Verification items for the finished model (mm, model axes). A direction names the side the tool comes from. Give positions to 0.01 mm unless a question says otherwise; leave off trailing zeros. Write each loop counter-clockwise with the first axis right and the second up, starting at its lowest first coordinate (ties: lowest second). Pieces come first, ordered by that corner, then holes. Notation, with made-up numbers: (79, 89) -> (121, 89) arc R30 cw to (121, 114) -> close; hole circle Ø10 at (8.25, 35.25). An arc over 180 degrees is marked (long way). Answer as CSV lines item,"result". Start each with the question number.
1) Material ranges on L1, parallel to Y at x = 5.5, z = 2.6; L2, parallel to Y at x = 5.5, z = 2.45; L3, parallel to Z at x = -4.5, y = 9, recorded low to high.
2) Sectioned sample at C-C on y = 14. Record the cut outline in (x, z), and give its area (3 significant figures).
3) Mould release check, pull along Y, two halves, no side actions. Record for faces 4 (the flat face through (5, 33, 1)), 5 (the flat face through (-4, 36, 1)), 6 (the flat face through (12, -11.5, 1)), 7 (the flat face through (6.25, 10, 1)): released by +Y, released by -Y, zero draft, split by the parting line, or undercut.
4) Gauge pin test, flat ends, axial feed: pin 1 Ø3.5 at (y, z) = (39.5, 1.5) entering from +X; pin 2 Ø12 at (x, y) = (9.5, 10.5) entering from +Z; pin 3 Ø2 at (y, z) = (2, 3.5) entering from +X; pin 4 Ø3 at (x, y) = (-2.5, 35) entering from -Z. Record the tip position at first contact, or that the pin passes through.
5) Tool access check on faces 1 (the flat face through (4, 42, 1)), 2 (the flat face through (6, 40, 2)), 3 (the cylindrical face through (6.63, -20.48, 2.01)). Record the directions out of +Z, -Z, +X, -X, +Y, -Y that give a thin tool (end or side, any length) a straight path to the whole face; none if there is none.
6) Sectioned sample at B-B on x = 10.75. Record the cut outline in (y, z), and give its area (3 significant figures).
7) Sectioned sample at A-A on y = -22.25. Record the cut outline in (x, z), and give its area (3 significant figures).
```python
from build123d import *

# Parameters (mm, degrees)
PAD_DEPTH    = 3
SKETCH001_R  = 1.5
PAD001_DEPTH = 6
SKETCH002_R  = 2.1
POCKET_DEPTH = 2
SKETCH003_R  = 3
PAD002_DEPTH = 3
FILLET_R     = 2.75


with BuildPart() as part:
    # Sketch → Pad (new body)
    with BuildSketch(Plane.XY):
        Polygon((-6.25, 33), (-6.25, -33), (17.25, -33), (17.25, -11.5), (6.25, -11.5), (6.25, 33), (4, 33), (4, 43), (-4, 43), (-4, 33), align=None)
    extrude(amount=PAD_DEPTH)

    # Sketch001 → Pad001 (join, symmetric)
    with BuildSketch(Plane.YZ):
        with Locations((40, 1.5)):
            Circle(SKETCH001_R)
    extrude(amount=PAD001_DEPTH, both=True)

    # Sketch002 (on Face5 of Pad001) → Pocket (cut)
    with BuildSketch(Plane.XY.offset(3)):
        with Locations((5.5, -22.25)):
            Circle(SKETCH002_R)
    extrude(amount=-POCKET_DEPTH, mode=Mode.SUBTRACT)

    # Sketch003 (on Face5 of Pocket) → Pad002 (join)
    with BuildSketch(Plane.XY.offset(3)):
        with Locations((0, 23)):
            Circle(SKETCH003_R)
    extrude(amount=PAD002_DEPTH)

    # Fillet
    fillet_edges = [part.edges().sort_by_distance(p)[0] for p in [
        (-3, 23, 6),
    ]]
    fillet(fillet_edges, radius=FILLET_R)


solid = part.part
```
Ans:
1,L1,"y = -33 to -24.35, -20.15 to 33, 38.98 to 41.02"
1,L2,"y = -33 to -24.35, -20.15 to 33, 38.84 to 41.16"
1,L3,"z = 0 to 3"
2,outline,"(-6.25, 0) -> (6.25, 0) -> (6.25, 3) -> (-6.25, 3) -> close"
2,area,"37.5 mm²"
3,face 4,"undercut"
3,face 5,"undercut"
3,face 6,"released by +Y"
3,face 7,"zero draft"
4,pin 1,"stops at x = 6"
4,pin 2,"stops at z = 3"
4,pin 3,"stops at x = 6.25"
4,pin 4,"stops at z = 0"
5,face 1,"+X, +Y"
5,face 2,"+Z, -Z, +X, +Y"
5,face 3,"+Z"
6,outline,"(-33, 0) -> (-11.5, 0) -> (-11.5, 3) -> (-33, 3) -> close"
6,area,"64.5 mm²"
7,outline,"(-6.25, 0) -> (17.25, 0) -> (17.25, 3) -> (7.6, 3) -> (7.6, 1) -> (3.4, 1) -> (3.4, 3) -> (-6.25, 3) -> close"
7,area,"62.1 mm²"
